```python
from build123d import *

# Parameters (mm, degrees)
SKETCH_1_R      = 7.4
SKETCH_1_R_2    = 0.95
EXTRUDE_1_DEPTH = 4
CHAMFER_1_SIZE  = 0.5


with BuildPart() as part:
    # Sketch 1 → Extrude 1 (new body)
    with BuildSketch(Plane(origin=(0, 0, 0), x_dir=(1, 0, 0), z_dir=(0, 1, 0))):
        with Locations(Location((0, 0, 0), (0, 0, 270))):
            Circle(SKETCH_1_R)
        with Locations(Location((2.7, 0, 0), (0, 0, 270))):
            Circle(SKETCH_1_R_2, mode=Mode.SUBTRACT)
        with Locations(Location((-1.3, 0, 0), (0, 0, 90))):
            Circle(SKETCH_1_R_2, mode=Mode.SUBTRACT)
    extrude(amount=EXTRUDE_1_DEPTH)

    # Chamfer 1
    chamfer_1_edges = [part.edges().sort_by_distance(p)[0] for p in [
        (0, 0, -7.4),
        (0, 4, -7.4),
        (2.7, 0, -0.95),
        (2.7, 4, -0.95),
        (-1.3, 0, 0.95),
        (-1.3, 4, 0.95),
    ]]
    chamfer(chamfer_1_edges, length=CHAMFER_1_SIZE)


solid = part.part
```
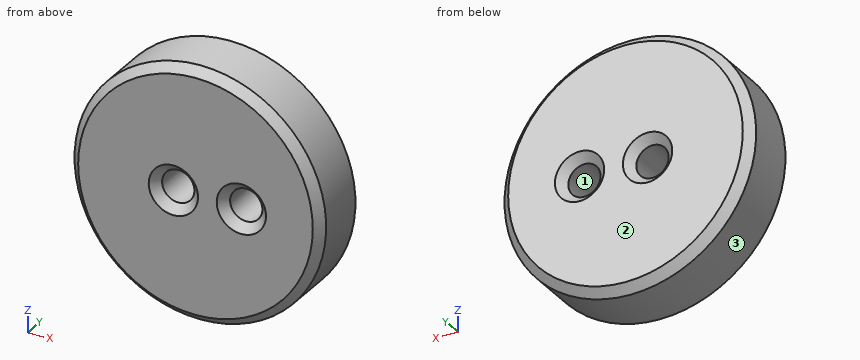
Read the model definition and answer for the solid it produces. Units are mm, in the model's axes. Face numbers are marked on the shaded views. Coordinates: 2 decimals unless noted, no trailing zeros. Write each loop counter-clockwise with the first axis right and the second up, starting at its lowest first coordinate (ties: lowest second). Pieces come first, ordered by that corner, then holes. Notation, with made-up numbers: (-15, -11) -> (5, -11) arc R23 ccw to (5, 20) -> close; hole circle Ø6 at (7, 82.5). An arc over 180 degrees is marked (long way). Answer as a JSON object with one key per item and string values.
Q1. Determine the mould class of the marked faces 1, 2 and 3 for opening direction X: pulls with the +X half, pulls with the -X half, needs draft (parallel to the pull), parting line crosses it, or undercut.
The answers:
{"face 1": "undercut", "face 2": "needs draft", "face 3": "parting line crosses it"}
Q2. The part is cut by section B-B on y = 1.4. Give the vertices of the cut face in (x, z).
The answers:
{"outline": "circle Ø14.8 at (0, 0); hole circle Ø1.9 at (-1.3, 0); hole circle Ø1.9 at (2.7, 0)"}
Q3. Consider line 1 (X direction, y = 1.45, z = 0); line 2 (X direction, y = 2.45, z = -0.5); line 3 (Z direction, x = 0.25, y = 1.8). Determine where each line is inside the solid, lowest interval first. Write a range as [from, to].
The answers:
{"line 1": "x = [-7.4, -2.25], [-0.35, 1.75], [3.65, 7.4]", "line 2": "x = [-7.38, -2.11], [-0.49, 1.89], [3.51, 7.38]", "line 3": "z = [-7.4, 7.4]"}
Q4. The part is cut by section A-A on z = 0. Give the vertices of the cut face in (x, y), then the cut area to 3 significant figures.
The answers:
{"outline": "(-7.4, 0.5) -> (-6.9, 0) -> (-2.75, 0) -> (-2.25, 0.5) -> (-2.25, 3.5) -> (-2.75, 4) -> (-6.9, 4) -> (-7.4, 3.5) -> close; (-0.35, 0.5) -> (0.15, 0) -> (1.25, 0) -> (1.75, 0.5) -> (1.75, 3.5) -> (1.25, 4) -> (0.15, 4) -> (-0.35, 3.5) -> close; (3.65, 0.5) -> (4.15, 0) -> (6.9, 0) -> (7.4, 0.5) -> (7.4, 3.5) -> (6.9, 4) -> (4.15, 4) -> (3.65, 3.5) -> close", "area": "42.5 mm2"}
Q5. Flat-ended cylindrical pins translate along their axes: pin 1 Ø2.5 at (x, z) = (2.7, 0) entering from +Y; pin 2 Ø1.5 at (x, z) = (-1.3, 0) entering from +Y. Find the tip coordinate at first contact, or state that the pin passes through.
The answers:
{"pin 1": "stops at y = 3.8", "pin 2": "passes through"}
